Can you work these out from the drawing? Everything is in mm from the part's minimum corner. A direction names the side the tool comes from. Coordinates: 2 decimals unless noted, no trailing zeros. Loops run counter-clockwise (first coordinate to the right, second up) from the corner with the lowest first, then second, coordinate; pieces in that order, holes last.
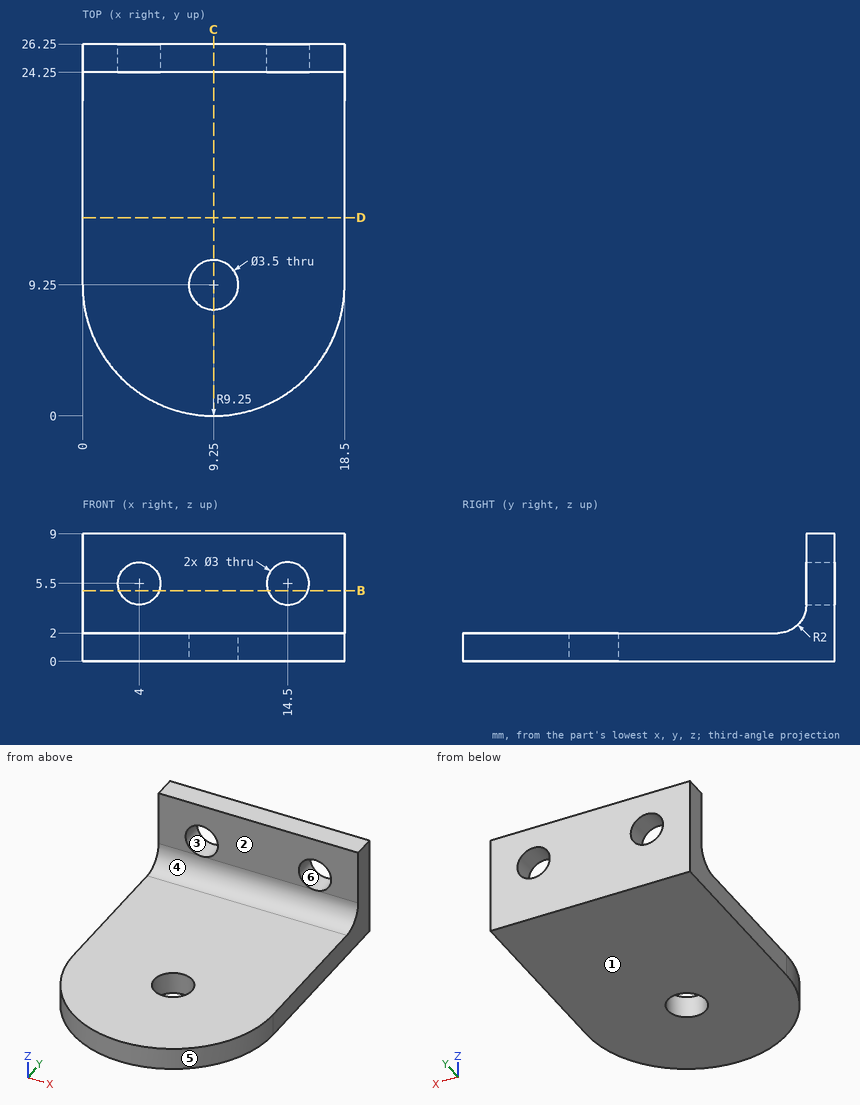
(1) We'd pull the mould along X, two halves only. Please class the marked faces 3, 4, 5 and 6: +X half, -X half, draft (parallel to the pull), parting line (faces both ways), or undercut.
Answers:
face 3: undercut
face 4: draft
face 5: parting line
face 6: undercut
(2) Imagine slicing it at D-D, the plane y = 14. Write out the boundary of the cut face in (x, z).
Answers:
outline: (0, 0) - (18.5, 0) - (18.5, 2) - (0, 2) - close
(3) For pin 1 (3.5 mm diameter, centred on x = 4, z = 5.5, fed in from -Y) (1 decimal); pin 2 (10 mm diameter, centred on x = 9.5, y = 8.5, fed in from +Z), each with a flat end and sliding along its axis, tell me the tip position at first contact or that it passes through.
Answers:
pin 1: stops at y = 24.2
pin 2: stops at z = 2
(4) Imagine slicing it at C-C, the plane x = 9.25. Write out the boundary of the cut face in (y, z).
Answers:
outline: (0, 0) - (7.5, 0) - (7.5, 2) - (0, 2) - close; (11, 0) - (26.25, 0) - (26.25, 9) - (24.25, 9) - (24.25, 4) arc R2 cw to (22.25, 2) - (11, 2) - close
(5) I need wall thicknesses on probe 1 along Z at (x, y) = (14.5, 25.3); probe 2 along Z at (x, y) = (10.25, 13); probe 3 along Y at (x, z) = (9.5, 4.75). Which ranges of each line are inside material? Lowest first, please.
Answers:
probe 1: z = 0 to 4, 7 to 9
probe 2: z = 0 to 2
probe 3: y = 24.25 to 26.25
(6) Which directions (+Z, -Z, +X, -X, +Y, -Y) give clear straight access to the entire face, cutting with the end or side of a thin tool? Please do the marked faces 1 and 2.
Answers:
face 1: -Z, +X, -X, +Y, -Y
face 2: +Z, +X, -X, -Y
(7) Imagine slicing it at B-B, the plane z = 5. State how many separate pieces and enclosed holes the cut face has.
Answers:
separate pieces: 3
enclosed holes: 0
